Source: CAD feature listing. Evaluate the final solid. Frame: model axes, mm. A direction names the side the tool comes from. Give positions to 0.01 mm unless a question says otherwise; leave off trailing zeros. Order: outer loops, then holes, each group sorted by start corner. A loop starts at its lowest first (then second) coordinate and runs counter-clockwise, first axis right, second up. Notation, with made-up numbers: M 62.25,3.25 L 83.25,3.25 A27 cw 83.25,31.25 Z; hole C 26,-18.75 d9. An arc over 180 degrees is marked long. Use CSV: the item, a comma, the result in double quotes. Start each with the question number.
Item 1: Section query A-A on z = -177. Return loops of the section in (x, y), and give its area (3 significant figures).
Item 2: Section query D-D on x = -106. Return loops of the section in (y, z).
Item 3: Ray query, probe 1 along X at (y, z) = (85, -177); probe 2 along Z at (x, y) = (-96.5, 43.5); probe 3 along Y at (x, z) = (-2, -86.5). Return the intervals inside material, ascending. Write a range as from..to.
Item 4: First-contact query: pin 1 (22.5 mm diameter, centred on x = -90, z = -62, fed in from -Y); pin 2 (18 mm diameter, centred on x = -90, z = -177, fed in from +Y). Flat tips, straight axial feed; report the tip coordinate or a pass-through.
Item 5: Pull-direction query (Z, two-part tool) for faces 4 (the face through (-95.2, 61.5, -2)), 5 (the face through (2, 57, -196)), 6 (the face through (2, 57, -200)); classes: +Z half, -Z half, draft (parallel to the pull), parting line (faces both ways), or undercut.
Item 6: Access query for faces 1 (the face through (1.75, 81.1, -5.804)), 2 (the face through (-5.911, 63.752, -1.972)), 3 (the face through (2, 52, 0)). Directions: +Z, -Z, +X, -X, +Y, -Y. A direction counts if a zero-diameter tool reaches every point of the face in a straight line with its end or side. Return the directions, or none.
Item 7: Section query B-B on x = -5. Return loops of the section in (y, z).
Item 8: Section query C-C on x = 80. Return loops of the section in (y, z).
from build123d import *

# Parameters (mm, degrees)
BASE_FLANGE1_DEPTH = 125
SKETCH6_R          = 7
CUT_EXTRUDE1_DEPTH = 10
SKETCH7_R          = 7
CUT_EXTRUDE2_DEPTH = 10


# Sheet-metal steps are written as plain solids
with BuildPart() as part:
    # Sketch1 → Base-Flange1 (new, symmetric)
    with BuildSketch(Plane(origin=(0, 0, 0), x_dir=(0, 0, -1), z_dir=(1, 0, 0))):
        with BuildLine():
            Line((0, 36.811428571), (0, 76.811428571))
            ThreePointArc((0, 76.811428571), (2.928932188, 83.882496383), (10, 86.811428571))
            Line((10, 86.811428571), (190, 86.811428571))
            ThreePointArc((190, 86.811428571), (197.071067812, 83.882496383), (200, 76.811428571))
            Line((200, 76.811428571), (200, 36.811428571))
            Line((200, 36.811428571), (196, 36.811428571))
            Line((196, 36.811428571), (196, 76.811428571))
            ThreePointArc((196, 76.811428571), (194.242640687, 81.054069259), (190, 82.811428571))
            Line((190, 82.811428571), (10, 82.811428571))
            ThreePointArc((10, 82.811428571), (5.757359313, 81.054069259), (4, 76.811428571))
            Line((4, 76.811428571), (4, 36.811428571))
            Line((4, 36.811428571), (0, 36.811428571))
        make_face()
    extrude(amount=BASE_FLANGE1_DEPTH, both=True)

    # Sketch6 → Cut-Extrude1 (cut)
    with BuildSketch(Plane(origin=(0, 86.811428571, 0), x_dir=(1, 0, 0), z_dir=(0, 1, 0))):
        with Locations(Location((-90, 177, 0), (0, 0, 270))):
            Circle(SKETCH6_R)
        with Locations(Location((80, 177, 0), (0, 0, 270))):
            Circle(SKETCH6_R)
        with Locations(Location((80, 62, 0), (0, 0, 270))):
            Circle(SKETCH6_R)
        with Locations(Location((-90, 62, 0), (0, 0, 270))):
            Circle(SKETCH6_R)
    extrude(amount=-CUT_EXTRUDE1_DEPTH, mode=Mode.SUBTRACT)

    # Sketch7 → Cut-Extrude2 (cut)
    with BuildSketch(Plane.XY):
        with Locations((-90, 56.811428571)):
            Circle(SKETCH7_R)
        with Locations((-5, 56.811428571)):
            Circle(SKETCH7_R)
        with Locations((80, 56.811428571)):
            Circle(SKETCH7_R)
    extrude(amount=-CUT_EXTRUDE2_DEPTH, mode=Mode.SUBTRACT)


solid = part.part
Verdict:
1,outline,"M -125,82.81 L -97,82.81 L -97,86.81 L -125,86.81 Z; M -83,82.81 L 73,82.81 L 73,86.81 L -83,86.81 Z; M 87,82.81 L 125,82.81 L 125,86.81 L 87,86.81 Z"
1,area,"888 mm2"
2,outline,"M 36.81,-200 L 76.81,-200 A10 ccw 86.81,-190 L 86.81,-10 A10 ccw 76.81,0 L 36.81,0 L 36.81,-4 L 76.81,-4 A6 cw 82.81,-10 L 82.81,-190 A6 cw 76.81,-196 L 36.81,-196 Z"
3,probe 1,"-125..-97, -83..73, 87..125"
3,probe 2,"-200..-196, -4..0"
3,probe 3,"82.81..86.81"
4,pin 1,"y = 82.81"
4,pin 2,"y = 86.81"
5,face 4,"draft"
5,face 5,"undercut"
5,face 6,"-Z half"
6,face 1,"+X, -X, -Y"
6,face 2,"+Z"
6,face 3,"+Z, +X, -X, +Y, -Y"
7,outline,"M 36.81,-200 L 76.81,-200 A10 ccw 86.81,-190 L 86.81,-10 A10 ccw 76.81,0 L 63.81,0 L 63.81,-4 L 76.81,-4 A6 cw 82.81,-10 L 82.81,-190 A6 cw 76.81,-196 L 36.81,-196 Z; M 36.81,-4 L 49.81,-4 L 49.81,0 L 36.81,0 Z"
8,outline,"M 36.81,-200 L 76.81,-200 A10 ccw 86.81,-190 L 86.81,-184 L 82.81,-184 L 82.81,-190 A6 cw 76.81,-196 L 36.81,-196 Z; M 36.81,-4 L 49.81,-4 L 49.81,0 L 36.81,0 Z; M 63.81,-4 L 76.81,-4 A6 cw 82.81,-10 L 82.81,-55 L 86.81,-55 L 86.81,-10 A10 ccw 76.81,0 L 63.81,0 Z; M 82.81,-170 L 86.81,-170 L 86.81,-69 L 82.81,-69 Z"
